from build123d import *

# Parameters (mm, degrees)
BOSS_EXTRUDE1_DEPTH           = 10
FILLET1_R                     = 3
CUT_EXTRUDE1_DEPTH            = 55.386
CHAMFER1_SIZE                 = 1.5
MIRROR3_START                 = -3.745316975
MIRROR3_DEPTH                 = 4.272002108
CSK_FOR_M4_SFHCS1_D           = 4
CSK_FOR_M4_SFHCS1_DEPTH       = 6.4
CSK_FOR_M4_SFHCS1_CSINK_D     = 6
CSK_FOR_M4_SFHCS1_CSINK_ANGLE = 90
CSK_FOR_M4_SFHCS2_D           = 4
CSK_FOR_M4_SFHCS2_CSINK_D     = 6
CSK_FOR_M4_SFHCS2_CSINK_ANGLE = 90
SKETCH7_R                     = 1.5
CUT_EXTRUDE2_DEPTH            = 24


# Read off the part's stored shape, not the designer's step: Mirror3
with BuildPart() as part:
    # Sketch1 → Boss-Extrude1 (new body)
    with BuildSketch(Plane(origin=(0, 0, 0), x_dir=(1, 0, 0), z_dir=(0, 1, 0))):
        with BuildLine():
            Line((-35.25, 0), (-35.25, -6.4))
            Line((-35.25, -6.4), (-22.25, -6.4))
            ThreePointArc((-22.25, -6.4), (-20.128679656, -7.278679656), (-19.25, -9.4))
            Line((-19.25, -9.4), (-19.25, -28.6))
            ThreePointArc((-19.25, -28.6), (-20.128679656, -30.721320344), (-22.25, -31.6))
            Line((-22.25, -31.6), (-35.25, -31.6))
            Line((-35.25, -31.6), (-35.25, -38))
            Line((-35.25, -38), (-5.75, -38))
            ThreePointArc((-5.75, -38), (-5.289009014, -37.946146786), (-4.852843875, -37.787487311))
            Line((-4.852843875, -37.787487311), (-0.384125597, -35.544596998))
            ThreePointArc((-0.384125597, -35.544596998), (0.230625744, -35.066359782), (0.616084961, -34.389564956))
            Line((0.616084961, -34.389564956), (1.30066574, -32.33582167))
            ThreePointArc((1.30066574, -32.33582167), (2.028611742, -31.34579265), (3.198032424, -30.968276939))
            Line((3.198032424, -30.968276939), (32.698032424, -30.968276939))
            ThreePointArc((32.698032424, -30.968276939), (33.642903174, -31.205546312), (34.363585035, -31.861057674))
            Line((34.363585035, -31.861057674), (35.193999483, -33.110222133))
            ThreePointArc((35.193999483, -33.110222133), (35.866740637, -33.73918414), (36.750000973, -34.000000252))
            Line((36.750000973, -34.000000252), (52.750000973, -34.000000252))
            Line((52.750000973, -34.000000252), (52.750000973, -4.000000252))
            Line((52.750000973, -4.000000252), (38.13600074, -4.000000252))
            ThreePointArc((38.13600074, -4.000000252), (36.996810987, -3.643851433), (36.263342318, -2.702246958))
            Line((36.263342318, -2.702246958), (35.25, 0))
            Line((35.25, 0), (-35.25, 0))
        make_face()
    extrude(amount=BOSS_EXTRUDE1_DEPTH)

    # Fillet1
    fillet1_edges = [part.edges().sort_by_distance(p)[0] for p in [
        (52.750000973, 0, 19.000000252),
        (-35.25, 0, 34.8),
        (-35.25, 0, 3.2),
        (-35.25, 10, 34.8),
        (52.750000973, 10, 19.000000252),
        (-35.25, 10, 3.2),
    ]]
    fillet(fillet1_edges, radius=FILLET1_R)

    # Sketch2 → Cut-Extrude1 (cut)
    with BuildSketch(Plane(origin=(38.13600074, 0, 0), x_dir=(0, 0, -1), z_dir=(1, 0, 0))):
        Polygon((-4.000000252, 10), (0, 10), (0, 8.5), align=None)
    extrude(amount=-CUT_EXTRUDE1_DEPTH, mode=Mode.SUBTRACT)

    # Chamfer1
    # the kernel refuses this chamfer: 1.5 mm, written as the material it adds along each edge
    with BuildSketch(Plane(origin=(-17.24999926, 7.145532803, -3.611912754), x_dir=(-0.027495876610586757, 0.9359751746095561, -0.35099066837171944), z_dir=(0, 0.3511234221997007, 0.9363291848398034))) as chamfer1_piece_1_section:
        Polygon((CHAMFER1_SIZE * 0.999621916911, -CHAMFER1_SIZE * 0.0274958766106), (-CHAMFER1_SIZE * 0.0274958766106, -CHAMFER1_SIZE * 0.999621916911), (0, 0), align=None)
    chamfer1_piece_1 = extrude(amount=11.987051072, mode=Mode.PRIVATE)
    chamfer1_piece_1 = split(chamfer1_piece_1, bisect_by=Plane(origin=(-16.68097762, 9.443284972, 0), z_dir=(0, 0, 1)), keep=Keep.TOP, mode=Mode.PRIVATE)
    chamfer1_piece_1 = split(chamfer1_piece_1, bisect_by=Plane(origin=(-16.68097762, 10, 1.484573502), z_dir=(0, -1, 0)), keep=Keep.TOP, mode=Mode.PRIVATE)
    add(chamfer1_piece_1)

    # Mirror3 outline → Mirror3 (cut)
    with BuildSketch(Plane(origin=(0, 0, 0), x_dir=(1, 0, 0), z_dir=(0, 0.3511234221997011, -0.9363291848398033)).offset(MIRROR3_START)):
        Polygon((-15.74999926, -1.404493777), (40, -1.404493777), (40, 2), (-19, 2), (-19, 1.845506963), align=None)
    extrude(amount=MIRROR3_DEPTH, mode=Mode.SUBTRACT)

    # CSK for M4 SFHCS1
    with Locations(Plane.XY.offset(6.4)):
        with Locations((-30.25, 5)):
            csk_for_m4_sfhcs1 = CounterSinkHole(CSK_FOR_M4_SFHCS1_D / 2, CSK_FOR_M4_SFHCS1_CSINK_D / 2, depth=CSK_FOR_M4_SFHCS1_DEPTH, counter_sink_angle=CSK_FOR_M4_SFHCS1_CSINK_ANGLE)

    # Mirror1: CSK for M4 SFHCS1 across plane
    add(csk_for_m4_sfhcs1.mirror(Plane.XY.offset(19)), mode=Mode.SUBTRACT)

    # CSK for M4 SFHCS2 (through all)
    with Locations(Plane.XY.offset(34.000000252)):
        with Locations((46.750000973, 5)):
            csk_for_m4_sfhcs2 = CounterSinkHole(CSK_FOR_M4_SFHCS2_D / 2, CSK_FOR_M4_SFHCS2_CSINK_D / 2, counter_sink_angle=CSK_FOR_M4_SFHCS2_CSINK_ANGLE)

    # Mirror2: CSK for M4 SFHCS2 across plane
    add(csk_for_m4_sfhcs2.mirror(Plane.XY.offset(19)), mode=Mode.SUBTRACT)

    # Sketch7 → Cut-Extrude2 (cut)
    with BuildSketch(Plane(origin=(0, 0, 0), x_dir=(-1, 0, 0), z_dir=(0, 0, -1))):
        with Locations((-31.25, 5)):
            Circle(SKETCH7_R)
        with Locations((-23.75, 5)):
            Circle(SKETCH7_R)
        with Locations((-16.25, 5)):
            Circle(SKETCH7_R)
        with Locations((-8.75, 5)):
            Circle(SKETCH7_R)
        with Locations((-1.25, 5)):
            Circle(SKETCH7_R)
        with Locations((6.25, 5)):
            Circle(SKETCH7_R)
        with Locations((13.75, 5)):
            Circle(SKETCH7_R)
    extrude(amount=-CUT_EXTRUDE2_DEPTH, mode=Mode.SUBTRACT)


solid = part.part
The listing builds one solid part. Answer for the finished solid, in the listing's coordinates (mm). A direction names the side the tool comes from. Round coordinates to 2 decimals unless told otherwise and drop trailing zeros. Write each loop counter-clockwise with the first axis right and the second up, starting at its lowest first coordinate (ties: lowest second). Pieces come first, ordered by that corner, then holes. Notation, with made-up numbers: M 24,18 L 34,18 A26 cw 34,51 Z; hole C 54.5,-6 d11. An arc over 180 degrees is marked long. Write each question's results on one line, items separated by ' | '. Start each with the question number.
Item 1: A cutting plane is placed at C-C on x = 31.25. Write down the section's boundary in (y, z), and give its area (3 significant figures).
Item 2: Flat-ended cylindrical pins translate along their axes: pin 1 Ø4 at (x, y) = (31.25, 5) entering from +Z; pin 2 Ø1 at (x, y) = (-0.5, 7) entering from +Z; pin 3 Ø5 at (y, z) = (4, 22) entering from -X. Find the tip coordinate at first contact, or state that the pin passes through.
Item 3: For faces 4 (the face through (31, 5, 24)), 5 (the face through (44, 3, 4)), 6 (the face through (-20.11, 4.93, 30.7)), determine the directions among +Z, -Z, +X, -X, +Y, -Y from which every point of the face is accessible in a straight line to the end or side of a thin tool.
Item 4: A cutting plane is placed at B-B on z = 12. State how many separate pieces and enclosed holes the cut face has, and give its area (3 significant figures).
Item 5: Straight lines are drawn through the part: L1, parallel to Y at x = -13.75, z = 17.5; L2, parallel to Z at x = -23, y = 7.25; L3, parallel to Z at x = 19.5, y = 2.75. For each, find the intervals that lie inside material, in ascending order. Write a range as [from, to].
Item 6: A cutting plane is placed at A-A on x = -30.25. Write down the section's boundary in (y, z).
Item 7: For a pull along Z with two mould halves and no side action, classify faces 1 (the face through (25.25, 5.07, 11.83)), 2 (the face through (-27, 5, 31.6)), 3 (the face through (-6, 5, 24)) as pulls with the +Z half, pulls with the -Z half, needs draft (parallel to the pull), parting line crosses it, or undercut.
Check sheet entries:
1) outline: M 0,4 L 1.5,0 L 3.5,0 L 3.5,24 L 6.5,24 L 6.5,0 L 8.5,0 L 10,4 L 10,30.97 L 0,30.97 Z | area: 232 mm²
2) pin 1: z = 31.05 | pin 2: z = 35.85 | pin 3: x = -19.25
3) face 4: -Z | face 5: -Z, +X, +Y, -Y | face 6: -X, +Y, -Y
4) separate pieces: 1 | enclosed holes: 8 | area: 654 mm²
5) L1: [0, 3.5], [6.5, 10] | L2: [0, 6.4], [31.6, 38] | L3: [0, 30.97]
6) outline: M 0,0 L 3,0 L 3,5.4 L 2,6.4 L 0,6.4 Z; M 0,31.6 L 2,31.6 L 3,32.6 L 3,38 L 0,38 Z; M 7,0 L 10,0 L 10,6.4 L 8,6.4 L 7,5.4 Z; M 7,32.6 L 8,31.6 L 10,31.6 L 10,38 L 7,38 Z
7) face 1: needs draft | face 2: undercut | face 3: pulls with the -Z half
